Can you work these out from the model? Positions are in its coordinate system, mm. Face numbers are marked on the shaded views. Coordinates: 2 decimals unless noted, no trailing zeros. Order: outer loops, then holes, each group sorted by start corner. A loop starts at its lowest first (then second) coordinate and runs counter-clockwise, first axis right, second up. Notation, with made-up numbers: M 1,13.5 L 35,13.5 A30 ccw 35,46.5 Z; hole C 6,48.5 d8. An arc over 180 degrees is marked long. Answer as a JSON object with one key per item and string values.
from build123d import *

# Parameters (mm, degrees)
SKETCH1_W           = 95.25
SKETCH1_H           = 95.25
SKETCH1_R           = 44.45
BOSS_EXTRUDE1_DEPTH = 215.9
SKETCH2_W           = 95.25
SKETCH2_H           = 95.25
BOSS_EXTRUDE2_DEPTH = 6.35
SKETCH4_W           = 95.25
SKETCH4_H           = 95.25
SKETCH4_R           = 44.45
BOSS_EXTRUDE4_DEPTH = 6.35


with BuildPart() as part:
    # Sketch1 → Boss-Extrude1 (new body)
    with BuildSketch(Plane(origin=(0, 0, 0), x_dir=(1, 0, 0), z_dir=(0, 1, 0))):
        with Locations((47.625, 47.625)):
            Rectangle(SKETCH1_W, SKETCH1_H)
        with Locations(Location((47.625, 47.625, 0), (0, 0, 270))):
            Circle(SKETCH1_R, mode=Mode.SUBTRACT)
    extrude(amount=BOSS_EXTRUDE1_DEPTH)

    # Sketch2 → Boss-Extrude2 (add)
    with BuildSketch(Plane.XZ):
        with Locations((47.625, -47.625)):
            Rectangle(SKETCH2_W, SKETCH2_H)
    extrude(amount=BOSS_EXTRUDE2_DEPTH)

    # Sketch4 → Boss-Extrude4 (add)
    with BuildSketch(Plane(origin=(0, 215.9, 0), x_dir=(1, 0, 0), z_dir=(0, 1, 0))):
        with Locations((47.625, 47.625)):
            Rectangle(SKETCH4_W, SKETCH4_H)
        with Locations(Location((47.625, 47.625, 0), (0, 0, 270))):
            Circle(SKETCH4_R, mode=Mode.SUBTRACT)
    extrude(amount=BOSS_EXTRUDE4_DEPTH)


solid = part.part
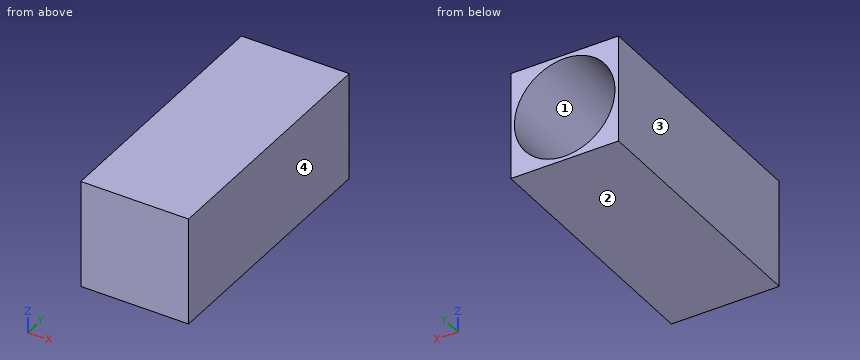
Item 1: I want a section at C-C, the plane y = 15. Write out the boundary of the cut face in (x, z) (3 decimals).
Answers follow:
{"outline": "M 0,-95.25 L 95.25,-95.25 L 95.25,0 L 0,0 Z; hole C 47.625,-47.625 d88.9"}
Item 2: I want a section at A-A, the plane x = 39. Write out the boundary of the cut face in (y, z), plus the area to 3 significant figures.
Answers follow:
{"outline": "M -6.35,-95.25 L 222.25,-95.25 L 222.25,-91.23 L 0,-91.23 L 0,-4.02 L 222.25,-4.02 L 222.25,0 L -6.35,0 Z", "area": "2,390 mm^2"}
Item 3: Please list where these lines run through material, in increasing order: line 1 (X direction, y = 53.5, z = -47); line 2 (Y direction, x = 8.5, z = -29); line 3 (X direction, y = 40, z = -68).
Answers follow:
{"line 1": "x = 0 to 3.18, 92.07 to 95.25", "line 2": "y = -6.35 to 0", "line 3": "x = 0 to 8.12, 87.13 to 95.25"}
Item 4: I want a section at B-B, the plane z = -58. Write out the boundary of the cut face in (x, y), plus the area to 3 significant figures.
Answers follow:
{"outline": "M 0,-6.35 L 95.25,-6.35 L 95.25,222.25 L 90.85,222.25 L 90.85,0 L 4.4,0 L 4.4,222.25 L 0,222.25 Z", "area": "2,560 mm^2"}
Item 5: If we mould it in two halves opening along X, with no side actions, what happens to the marked faces 1, 2, 3 and 4? For each: pulls with the +X half, pulls with the -X half, needs draft (parallel to the pull), parting line crosses it, or undercut.
Answers follow:
{"face 1": "undercut", "face 2": "needs draft", "face 3": "pulls with the -X half", "face 4": "pulls with the +X half"}
